from build123d import *

# Parameters (mm, degrees)
F0_R     = 12.7
F1_DEPTH = 25.4


with BuildPart() as f1:
    # F0 (on Front) → F1 (new body)
    with BuildSketch(Plane.XZ):
        with BuildLine():
            ThreePointArc((0, -44.45), (-44.45, 0), (0, 44.45))
            Line((0, 44.45), (0, 63.5))
            ThreePointArc((0, 63.5), (-25.116623, 58.321568), (-46.136719, 43.630874))
            ThreePointArc((-46.136719, 43.630874), (-59.347524, 34.564632), (-75.117614, 31.731545))
            ThreePointArc((-75.117614, 31.731545), (-107.95, 0), (-75.117614, -31.731545))
            ThreePointArc((-75.117614, -31.731545), (-59.347524, -34.564632), (-46.136719, -43.630874))
            ThreePointArc((-46.136719, -43.630874), (-25.116623, -58.321568), (0, -63.5))
            Line((0, -63.5), (0, -44.45))
        make_face()
        with Locations((-76.2, 0)):
            Circle(F0_R, mode=Mode.SUBTRACT)
        with BuildLine():
            ThreePointArc((0, 44.45), (31.430896, 31.430896), (44.45, 0))
            ThreePointArc((44.45, 0), (31.430896, -31.430896), (0, -44.45))
            Line((0, -44.45), (0, -63.5))
            ThreePointArc((0, -63.5), (25.116623, -58.321568), (46.136719, -43.630874))
            ThreePointArc((46.136719, -43.630874), (59.347524, -34.564632), (75.117614, -31.731545))
            ThreePointArc((75.117614, -31.731545), (107.95, 0), (75.117614, 31.731545))
            ThreePointArc((75.117614, 31.731545), (59.347524, 34.564632), (46.136719, 43.630874))
            ThreePointArc((46.136719, 43.630874), (25.116623, 58.321568), (0, 63.5))
            Line((0, 63.5), (0, 44.45))
        make_face()
        with Locations((76.2, 0)):
            Circle(F0_R, mode=Mode.SUBTRACT)
    extrude(amount=F1_DEPTH)


solid = f1.part
Geometry: final body of the model. Coordinates: model frame, mm. Give positions to 0.01 mm unless a question says otherwise; leave off trailing zeros. Write each loop counter-clockwise with the first axis right and the second up, starting at its lowest first coordinate (ties: lowest second). Pieces come first, ordered by that corner, then holes. Notation, with made-up numbers: M -10,-7.75 L 2,-7.75 A18 ccw 2,-3.75 Z; hole C -3,34 d3. An arc over 180 degrees is marked long. Answer in a Markdown table with one row per item. Add a question column.
(1) Section A-A on x = -84.5. Return loops of the section in (y, z).
(2) First-contact query: pin 1 (1 mm diameter, centred on x = 40, y = -12, fed in from +Z); pin 2 (10 mm diameter, centred on y = -4.5, z = -2.5, fed in from +X); pin 3 (8 mm diameter, centred on x = 59, y = -13, fed in from -Z). Flat tips, straight axial feed; report the tip coordinate or a pass-through.
(3) Mould query, pull axis Z, two halves, no side actions, for faces 1 (the cylindrical face through (63.512, -12.522, 0.558)), 2 (the cylindrical face through (-59.14, -12.52, 34.65)), 3 (the flat face through (46, -25.4, 1)). Classes: +Z half, -Z half, draft (parallel to the pull), parting line (faces both ways), or undercut.
(4) Section D-D on x = -52.5. Return loops of the section in (y, z), and give its area (3 significant figures).
(5) Section B-B on y = -22. Return loops of the section in (x, z).
(6) Section C-C on z = 52.5. Return loops of the section in (x, y), and give its area (3 significant figures).
(7) Ray query, line 1 (X direction, y = -3, z = 9); line 2 (X direction, y = -22, z = -55); line 3 (Z direction, x = -76.2, y = -15). Return the intervals inside material, ascending.
Result set:
| question | item | result |
|---|---|---|
| 1 | outline | M -25.4,-30.65 L 0,-30.65 L 0,-9.61 L -25.4,-9.61 Z; M -25.4,9.61 L 0,9.61 L 0,30.65 L -25.4,30.65 Z |
| 2 | pin 1 | stops at z = 49.72 |
| 2 | pin 2 | stops at x = 107.95 |
| 2 | pin 3 | stops at z = -36.68 |
| 3 | face 1 | undercut |
| 3 | face 2 | +Z half |
| 3 | face 3 | draft |
| 4 | outline | M -25.4,-38.23 L 0,-38.23 L 0,38.23 L -25.4,38.23 Z |
| 4 | area | 1,940 mm^2 |
| 5 | outline | M -75.12,-31.73 A38.1 cw -46.14,-43.63 A63.5 ccw 0,-63.5 A63.5 ccw 46.14,-43.63 A38.1 cw 75.12,-31.73 A31.75 ccw long 75.12,31.73 A38.1 cw 46.14,43.63 A63.5 ccw 0,63.5 A63.5 ccw -46.14,43.63 A38.1 cw -75.12,31.73 A31.75 ccw long Z; hole C -76.2,0 d25.4; hole M 0,-44.45 A44.45 ccw 44.45,0 A44.45 ccw 0,44.45 A44.45 ccw Z; hole C 76.2,0 d25.4 |
| 6 | outline | M -35.72,-25.4 L 35.72,-25.4 L 35.72,0 L -35.72,0 Z |
| 6 | area | 1,810 mm^2 |
| 7 | line 1 | x = -106.65 to -85.16, -67.24 to -43.53, 43.53 to 67.24, 85.16 to 106.65 |
| 7 | line 2 | x = -31.74 to 31.74 |
| 7 | line 3 | z = -31.75 to -12.7, 12.7 to 31.75 |
